Source: CAD feature listing. Evaluate the final solid. Frame: model axes, mm. A direction names the side the tool comes from. Round coordinates to 2 decimals unless told otherwise and drop trailing zeros. Write each loop counter-clockwise with the first axis right and the second up, starting at its lowest first coordinate (ties: lowest second). Pieces come first, ordered by that corner, then holes. Notation, with made-up numbers: M 47,46.5 L 62,46.5 A17 ccw 62,62.5 Z; hole C 24,-26.75 d1. An arc over 180 degrees is marked long. Use a Markdown table: item, result.
```python
from build123d import *

# Parameters (mm, degrees)
SKETCH_1_R          = 6
SKETCH_1_R_2        = 2.05
SKETCH_1_R_3        = 1.55
EXTRUDE_1_DEPTH     = 5
FILLET_1_R          = 40
CUT_EXTRUDE_1_DEPTH = 249.231362274
CUT_EXTRUDE_2_DEPTH = 249.231362274


with BuildPart() as part:
    # 草图1 → 凸台-拉伸1 (new body)
    # profile 1 of 6: a face of its own
    with BuildSketch(Plane.XY):
        with BuildLine():
            Line((6, 0), (6, 148.536084387))
            Line((6, 148.536084387), (5.143034079, 147.109821936))
            ThreePointArc((5.143034079, 147.109821936), (-1.603401935, 144.418209427), (-6, 150.2))
            Line((-6, 150.2), (-6, 0))
            ThreePointArc((-6, 0), (0, 6), (6, 0))
        make_face()
    # profile 2 of 6: a face of its own
    with BuildSketch(Plane.XY):
        Circle(SKETCH_1_R)
        Circle(SKETCH_1_R_2, mode=Mode.SUBTRACT)
    # profile 3 of 6: a face of its own
    with BuildSketch(Plane.XY):
        with BuildLine():
            Line((6, 148.536084387), (56.388486973, 232.398470405))
            ThreePointArc((56.388486973, 232.398470405), (48.155274831, 230.34561439), (46.102418816, 238.578826533))
            Line((46.102418816, 238.578826533), (-5.143034079, 153.290178064))
            ThreePointArc((-5.143034079, 153.290178064), (1.603401935, 155.981790573), (6, 150.2))
            Line((6, 150.2), (6, 148.536084387))
        make_face()
    # profile 4 of 6: a face of its own
    with BuildSketch(Plane.XY):
        with Locations((51.245452895, 235.488648469)):
            Circle(SKETCH_1_R)
        with Locations((51.245452895, 235.488648469)):
            Circle(SKETCH_1_R_3, mode=Mode.SUBTRACT)
    # profile 5 of 6: a face of its own
    with BuildSketch(Plane.XY):
        with Locations((0, 150.2)):
            Circle(SKETCH_1_R)
        with Locations((0, 150.2)):
            Circle(SKETCH_1_R_3, mode=Mode.SUBTRACT)
    # profile 6 of 6: a face of its own
    with BuildSketch(Plane.XY):
        with BuildLine():
            Line((5.143034079, 147.109821936), (6, 148.536084387))
            Line((6, 148.536084387), (6, 150.2))
            ThreePointArc((6, 150.2), (5.781790573, 148.596598065), (5.143034079, 147.109821936))
        make_face()
    extrude(amount=EXTRUDE_1_DEPTH)

    # 圆角1
    fillet_1_edges = [part.edges().sort_by_distance(p)[0] for p in [
        (6, 148.536084387, 2.5),
    ]]
    fillet(fillet_1_edges, radius=FILLET_1_R)

    # 草图3 → 切除-拉伸1 (cut, through all)
    with BuildSketch(Plane.XY.offset(5)):
        with BuildLine():
            Line((2.5, 135.2), (2.5, 15))
            ThreePointArc((2.5, 15), (0, 12.5), (-2.5, 15))
            Line((-2.5, 15), (-2.5, 135.2))
            ThreePointArc((-2.5, 135.2), (0, 137.7), (2.5, 135.2))
        make_face()
    extrude(amount=-CUT_EXTRUDE_1_DEPTH, mode=Mode.SUBTRACT)

    # 草图4 → 切除-拉伸2 (cut, through all)
    with BuildSketch(Plane.XY.offset(5)):
        with BuildLine():
            Line((47.208027633, 223.915006118), (8.323286994, 159.198493964))
            ThreePointArc((8.323286994, 159.198493964), (4.892781935, 158.343137291), (4.037425262, 161.77364235))
            Line((4.037425262, 161.77364235), (42.922165901, 226.490154505))
            ThreePointArc((42.922165901, 226.490154505), (46.35267096, 227.345511178), (47.208027633, 223.915006118))
        make_face()
    extrude(amount=-CUT_EXTRUDE_2_DEPTH, mode=Mode.SUBTRACT)


solid = part.part
```
Q1. Line query: L1, parallel to X at y = 89.5, z = 2.8; L2, parallel to Y at x = 0, z = 3.85; L3, parallel to Y at x = -1, z = 1.5. Output: solid intervals per line, ascending.
Results are:
| item | result |
|---|---|
| L1 | -6 to -2.5, 2.5 to 6 |
| L2 | -6 to -2.05, 2.05 to 12.5, 137.7 to 148.65, 151.75 to 161.85 |
| L3 | -5.92 to -1.79, 1.79 to 12.71, 137.49 to 149.02, 151.38 to 160.19 |
Q2. Section C-C on z = 2.45. Give the number of separate pieces and of enclosed holes in the cut face, plus the area to 3 significant figures.
Results are:
| item | result |
|---|---|
| separate pieces | 1 |
| enclosed holes | 5 |
| area | 2,070 mm^2 |
Q3. Section A-A on y = 98.5. Return loops of the section in (x, z), plus the area to 3 significant figures.
Results are:
| item | result |
|---|---|
| outline | M -6,0 L -2.5,0 L -2.5,5 L -6,5 Z; M 2.5,0 L 6,0 L 6,5 L 2.5,5 Z |
| area | 35.0 mm^2 |
Q4. Mould query, pull axis Y, two halves, no side actions, for faces 3 (the cylindrical face through (0.1, 12.5, 2.5)), 4 (the cylindrical face through (0, -6, 2)), 5 (the flat face through (6, 68, 2)). Classes: +Y half, -Y half, draft (parallel to the pull), parting line (faces both ways), or undercut.
Results are:
| item | result |
|---|---|
| face 3 | undercut |
| face 4 | -Y half |
| face 5 | draft |
Q5. First-contact query: pin 1 Ø3 at (x, y) = (0, 150.2) entering from +Z; pin 2 Ø2 at (x, z) = (24.5, 2.5) entering from -Y. Flat tips, straight axial feed; report the tip coordinate or a pass-through.
Results are:
| item | result |
|---|---|
| pin 1 | through |
| pin 2 | y = 177.66 |
Q6. Reachability of faces 1 (the cylindrical face through (-0.1, 137.7, 2.5)), 2 (the cylindrical face through (7.5, 148.3, 2.5)) from +Z, -Z, +X, -X, +Y, -Y: full face, straight path, thin tool, end or side. Return the list, or none.
Results are:
| item | result |
|---|---|
| face 1 | +Z, -Z |
| face 2 | +Z, -Z, +X, -Y |
Q7. Section B-B on x = 37.5. Return loops of the section in (y, z), plus the area to 3 significant figures.
Results are:
| item | result |
|---|---|
| outline | M 200.96,0 L 207.76,0 L 207.76,5 L 200.96,5 Z; M 217.47,0 L 224.26,0 L 224.26,5 L 217.47,5 Z |
| area | 68.0 mm^2 |
